Read the model definition and answer for the solid it produces. Units are mm, in the model's axes. Round coordinates to 2 decimals unless told otherwise and drop trailing zeros. Order: outer loops, then holes, each group sorted by start corner. A loop starts at its lowest first (then second) coordinate and runs counter-clockwise, first axis right, second up. Notation, with made-up numbers: (-2.5, 62) -> (9.5, 62) arc R22 cw to (9.5, 83) -> close; hole circle Ø10 at (-39, 29). An arc over 180 degrees is marked (long way). Answer as a JSON object with one key per item and string values. Group by question number.
Item 1: Consider probe 1 along X at (y, z) = (2.05, 75); probe 2 along Z at (x, y) = (115, 2); probe 3 along Y at (x, z) = (90, -71.6). Determine where each line is inside the solid, lowest interval first. Write a range as from..to.
Item 2: Given P1, Ø5.5, axis at x = 115, z = -75, coming from the -Y side; P2, Ø5.5, axis at x = 90, y = -6, coming from the -Z side; P3, Ø1.5, axis at y = -18.5, z = 72.5, coming from the +X side; P4, Ø3, axis at x = 80, z = -20, coming from the +Y side, each flat-ended and moving along its own axis, determine where each tip first touches the part or whether it passes through.
Item 3: Section B-B, the plane z = 0 is taken. Write down the section's boundary in (x, y), plus the area to 3 significant figures.
Item 4: Section A-A, the plane x = 31 is taken. Write down the section's boundary in (y, z).
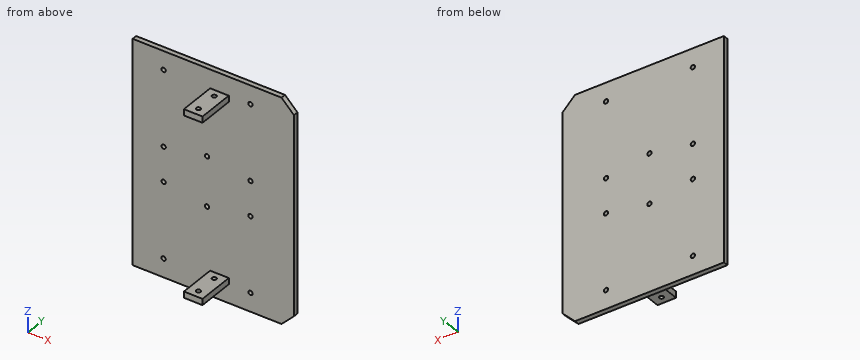
from build123d import *

# Parameters (mm, degrees)
SKETCH1_W               = 300
SKETCH1_H               = 180
MAIN_BODY_DEPTH         = 4
FILLET1_R               = 10
CHAMFER1_SIZE           = 10
SKETCH2_R               = 1.75
BATTERIES_HOLES_DEPTH   = 15
SKETCH5_R               = 1.75
SKETCH5_W               = 15
SKETCH5_H               = 10
L298N_HOLES_DEPTH       = 15
SKETCH6_R               = 1.75
LM2596_HOLES_DEPTH      = 15
SKETCH7_R               = 1.55
ESP32_HOLES_DEPTH       = 15
SKETCH8_R               = 1.75
PCB_SENSORS_HOLES_DEPTH = 15
SKETCH9_W               = 15
SKETCH9_H               = 5
WHEELS_LEGS_DEPTH       = 30
SKETCH10_R              = 1.75
MOTOR_HOLES_DEPTH       = 300
SKETCH11_R              = 1.75
SKETCH11_W              = 30
SKETCH11_H              = 20
SENSORS_HOLES_DEPTH     = 15
SKETCH13_W              = 40
SKETCH13_H              = 75
CUT_EXTRUDE2_DEPTH      = 10
FILLET2_R               = 10
SKETCH12_R              = 1.75
CUT_EXTRUDE3_DEPTH      = 10
SKETCH14_W              = 212.137898895
SKETCH14_H              = 97.482026014
CUT_EXTRUDE4_DEPTH      = 200


with BuildPart() as part:
    # Sketch1 → Main Body (new body)
    with BuildSketch(Plane(origin=(0, 0, 0), x_dir=(1, 0, 0), z_dir=(0, 1, 0))):
        Rectangle(SKETCH1_W, SKETCH1_H)
    extrude(amount=MAIN_BODY_DEPTH)

    # Fillet1
    fillet1_edges = [part.edges().sort_by_distance(p)[0] for p in [
        (-150, 2, 90),
        (-150, 2, -90),
    ]]
    fillet(fillet1_edges, radius=FILLET1_R)

    # Chamfer1
    chamfer1_edges = [part.edges().sort_by_distance(p)[0] for p in [
        (150, 2, 90),
        (150, 2, -90),
    ]]
    chamfer(chamfer1_edges, length=CHAMFER1_SIZE)

    # Sketch2 → Batteries holes (cut)
    with BuildSketch(Plane(origin=(0, 4, 0), x_dir=(1, 0, 0), z_dir=(0, 1, 0))):
        with Locations(Location((115, 75, 0), (0, 0, 270))):
            Circle(SKETCH2_R)
        with Locations(Location((115, 14, 0), (0, 0, 270))):
            Circle(SKETCH2_R)
        with Locations(Location((115, -14, 0), (0, 0, 90))):
            Circle(SKETCH2_R)
        with Locations(Location((115, -75, 0), (0, 0, 90))):
            Circle(SKETCH2_R)
        with Locations(Location((45, -75, 0), (0, 0, 270))):
            Circle(SKETCH2_R)
        with Locations(Location((45, -14, 0), (0, 0, 270))):
            Circle(SKETCH2_R)
        with Locations(Location((45, 14, 0), (0, 0, 90))):
            Circle(SKETCH2_R)
        with Locations(Location((45, 75, 0), (0, 0, 90))):
            Circle(SKETCH2_R)
    extrude(amount=-BATTERIES_HOLES_DEPTH, mode=Mode.SUBTRACT)

    # Sketch5 → L298N holes (cut)
    with BuildSketch(Plane(origin=(0, 4, 0), x_dir=(1, 0, 0), z_dir=(0, 1, 0))):
        with Locations(Location((-37, 18.5, 0), (0, 0, 270))):
            Circle(SKETCH5_R)
        with Locations(Location((0, 18.5, 0), (0, 0, 270))):
            Circle(SKETCH5_R)
        with Locations(Location((-37, -18.5, 0), (0, 0, 270))):
            Circle(SKETCH5_R)
        with Locations(Location((0, -18.5, 0), (0, 0, 270))):
            Circle(SKETCH5_R)
        with Locations((-12.5, -38.5)):
            Rectangle(SKETCH5_W, SKETCH5_H)
        with Locations((-12.5, 38.5)):
            Rectangle(SKETCH5_W, SKETCH5_H)
    extrude(amount=-L298N_HOLES_DEPTH, mode=Mode.SUBTRACT)

    # Sketch6 → LM2596 holes (cut)
    with BuildSketch(Plane(origin=(0, 4, 0), x_dir=(1, 0, 0), z_dir=(0, 1, 0))):
        with Locations(Location((-33, 70, 0), (0, 0, 270))):
            Circle(SKETCH6_R)
        with Locations(Location((-3, 54, 0), (0, 0, 270))):
            Circle(SKETCH6_R)
        with Locations(Location((-33, -54, 0), (0, 0, 270))):
            Circle(SKETCH6_R)
        with Locations(Location((-3, -70, 0), (0, 0, 270))):
            Circle(SKETCH6_R)
    extrude(amount=-LM2596_HOLES_DEPTH, mode=Mode.SUBTRACT)

    # Sketch7 → ESP32 holes (cut)
    with BuildSketch(Plane(origin=(0, 4, 0), x_dir=(1, 0, 0), z_dir=(0, 1, 0))):
        with Locations(Location((-73, 65, 0), (0, 0, 270))):
            Circle(SKETCH7_R)
        with Locations(Location((-73, 19, 0), (0, 0, 270))):
            Circle(SKETCH7_R)
        with Locations(Location((-91, 19, 0), (0, 0, 270))):
            Circle(SKETCH7_R)
    extrude(amount=-ESP32_HOLES_DEPTH, mode=Mode.SUBTRACT)

    # Sketch8 → PCB sensors holes (cut)
    with BuildSketch(Plane(origin=(0, 4, 0), x_dir=(1, 0, 0), z_dir=(0, 1, 0))):
        with Locations(Location((-103, -54, 0), (0, 0, 270))):
            Circle(SKETCH8_R)
        with Locations(Location((-68, -54, 0), (0, 0, 90))):
            Circle(SKETCH8_R)
    extrude(amount=-PCB_SENSORS_HOLES_DEPTH, mode=Mode.SUBTRACT)

    # Sketch9 → Wheels legs (add)
    with BuildSketch(Plane.XZ):
        with Locations((-90, 72.5)):
            Rectangle(SKETCH9_W, SKETCH9_H)
        with Locations((90, 72.5)):
            Rectangle(SKETCH9_W, SKETCH9_H)
        with Locations((90, -72.5)):
            Rectangle(SKETCH9_W, SKETCH9_H)
        with Locations((-90, -72.5)):
            Rectangle(SKETCH9_W, SKETCH9_H)
    extrude(amount=WHEELS_LEGS_DEPTH)

    # Sketch10 → Motor holes (cut)
    with BuildSketch(Plane.XY.offset(75)):
        with Locations((-90, -24)):
            Circle(SKETCH10_R)
        with Locations((-90, -6)):
            Circle(SKETCH10_R)
        with Locations((90, -6)):
            Circle(SKETCH10_R)
        with Locations((90, -24)):
            Circle(SKETCH10_R)
    extrude(amount=-MOTOR_HOLES_DEPTH, mode=Mode.SUBTRACT)

    # Sketch11 → Sensors holes (cut)
    with BuildSketch(Plane(origin=(0, 4, 0), x_dir=(1, 0, 0), z_dir=(0, 1, 0))):
        with Locations(Location((-140, 10, 0), (0, 0, 270))):
            Circle(SKETCH11_R)
        with Locations(Location((-125, 10, 0), (0, 0, 270))):
            Circle(SKETCH11_R)
        with Locations(Location((-125, 30, 0), (0, 0, 90))):
            Circle(SKETCH11_R)
        with Locations(Location((-140, 30, 0), (0, 0, 90))):
            Circle(SKETCH11_R)
        with Locations(Location((-125, -30, 0), (0, 0, 270))):
            Circle(SKETCH11_R)
        with Locations(Location((-140, -30, 0), (0, 0, 270))):
            Circle(SKETCH11_R)
        with Locations(Location((-125, -10, 0), (0, 0, 90))):
            Circle(SKETCH11_R)
        with Locations(Location((-140, -10, 0), (0, 0, 90))):
            Circle(SKETCH11_R)
        with Locations((-85, 0)):
            Rectangle(SKETCH11_W, SKETCH11_H)
    extrude(amount=-SENSORS_HOLES_DEPTH, mode=Mode.SUBTRACT)

    # Sketch13 → Cut-Extrude2 (cut)
    with BuildSketch(Plane.XZ):
        with Locations((-133, 75.5)):
            Rectangle(SKETCH13_W, SKETCH13_H)
        with Locations((-133, -75.5)):
            Rectangle(SKETCH13_W, SKETCH13_H)
    extrude(amount=-CUT_EXTRUDE2_DEPTH, mode=Mode.SUBTRACT)

    # Fillet2
    fillet2_edges = [part.edges().sort_by_distance(p)[0] for p in [
        (-113, 2, 90),
        (-150, 2, 38),
        (-113, 2, 38),
        (-113, 2, -90),
        (-113, 2, -38),
        (-150, 2, -38),
    ]]
    fillet(fillet2_edges, radius=FILLET2_R)

    # Sketch12 → Cut-Extrude3 (cut)
    with BuildSketch(Plane(origin=(0, 4, 0), x_dir=(1, 0, 0), z_dir=(0, 1, 0))):
        with Locations(Location((80, 20, 0), (0, 0, 270))):
            Circle(SKETCH12_R)
        with Locations(Location((80, -20, 0), (0, 0, 90))):
            Circle(SKETCH12_R)
        with Locations(Location((-20, -20, 0), (0, 0, 270))):
            Circle(SKETCH12_R)
        with Locations(Location((-20, 20, 0), (0, 0, 90))):
            Circle(SKETCH12_R)
    extrude(amount=-CUT_EXTRUDE3_DEPTH, mode=Mode.SUBTRACT)

    # Sketch14 → Cut-Extrude4 (cut)
    with BuildSketch(Plane.ZY.offset(-20)):
        with Locations((1.063142902, -9.465230627)):
            Rectangle(SKETCH14_W, SKETCH14_H)
    extrude(amount=CUT_EXTRUDE4_DEPTH, mode=Mode.SUBTRACT)


solid = part.part
Values found:
{
 "1": {"probe 1": "20..43.25, 46.75..113.25, 116.75..150", "probe 2": "-90..-76.75, -73.25..-15.75, -12.25..12.25, 15.75..73.25, 76.75..90", "probe 3": "-30..-25.75, -22.25..-7.75, -4.25..4"},
 "2": {"P1": "y = 0", "P2": "z = -75", "P3": "x = 97.5", "P4": "through"},
 "3": {"outline": "(20, 0) -> (150, 0) -> (150, 4) -> (20, 4) -> close", "area": "520 mm2"},
 "4": {"outline": "(0, -90) -> (4, -90) -> (4, 90) -> (0, 90) -> close"}
}
